Check sheet for the modelled part. Datum: model origin and axes. Units: mm. Give positions to 0.01 mm unless a question says otherwise; leave off trailing zeros. Loops run counter-clockwise (first coordinate to the right, second up) from the corner with the lowest first, then second, coordinate; pieces in that order, holes last. Notation, with made-up numbers: (-15, 10.5) -> (16, 10.5) arc R29 ccw to (16, 49.5) -> close; hole circle Ø4 at (4.5, 9). An arc over 180 degrees is marked (long way). Answer as CSV lines item,"result". Start each with the question number.
(1) Release check for a two-part mould opening along Y. For faces 1 (the face through (0.02, -6.59, 1.46)), 2 (the face through (0.02, 0.24, -20.64)), 3 (the face through (0.022, -16.642, -18.083)), 4 (the face through (-1.588, 5, -5)) record: pulls with the +Y half, pulls with the -Y half, needs draft (parallel to the pull), parting line crosses it, or undercut.
(2) Material ranges on line 1 (Y direction, x = -0.2, z = 0); line 2 (Z direction, x = 0.7, y = 5); line 3 (Y direction, x = 1, z = 4.5), recorded low to high. Write a range as from..to.
(3) Section check A-A on y = 0. Enter the section's corners in (x, z).
(4) Section check D-D on z = -13. Enter the section's corners in (x, y).
(5) Gauge pin test, flat end, axial feed: pin 1 Ø1.5 at (x, z) = (-1, -22.5) entering from -Y. Record the tip position at first contact, or that the pin passes through.
from build123d import *

# Parameters (mm, degrees)
SKETCH1_R             = 6.749999962
BOSS_EXTRUDE1_DEPTH   = 1.5875
FILLET1_R             = 0.508
FILLET2_R             = 0.508
M12_CLEARANCE_HOLE1_D = 13.5


with BuildPart() as part:
    # Sketch1 → Boss-Extrude1 (new, symmetric)
    # profile 1 of 2: a face of its own
    with BuildSketch(Plane(origin=(0, 0, 0), x_dir=(0, 0, -1), z_dir=(1, 0, 0))):
        with BuildLine():
            Line((33.3375, -12.7), (5.163771309, -19.981037814))
            ThreePointArc((5.163771309, -19.981037814), (-20.6375, 0), (5.163771309, 19.981037814))
            Line((5.163771309, 19.981037814), (33.3375, 12.7))
            ThreePointArc((33.3375, 12.7), (20.6375, 0), (33.3375, -12.7))
        make_face()
        Circle(SKETCH1_R, mode=Mode.SUBTRACT)
    # profile 2 of 2: a face of its own
    with BuildSketch(Plane(origin=(0, 0, 0), x_dir=(0, 0, -1), z_dir=(1, 0, 0))):
        Circle(SKETCH1_R)
    extrude(amount=BOSS_EXTRUDE1_DEPTH, both=True)

    # Fillet1
    fillet1_edges = [part.edges().sort_by_distance(p)[0] for p in [
        (0, -12.7, -33.3375),
    ]]
    fillet(fillet1_edges, radius=FILLET1_R)

    # Fillet2
    fillet2_edges = [part.edges().sort_by_distance(p)[0] for p in [
        (0, 12.7, -33.3375),
    ]]
    fillet(fillet2_edges, radius=FILLET2_R)

    # M12 Clearance Hole1 (through all)
    with Locations(Plane.ZY.offset(1.5875)):
        with Locations((0, 0)):
            Hole(M12_CLEARANCE_HOLE1_D / 2)


solid = part.part
Working result:
1,face 1,"undercut"
1,face 2,"undercut"
1,face 3,"pulls with the -Y half"
1,face 4,"needs draft"
2,line 1,"y = -20.64..-6.75, 6.75..20.64"
2,line 2,"z = -21.66..-4.53, 4.53..20.02"
2,line 3,"y = -20.14..-5.03, 5.03..20.14"
3,outline,"(-1.59, -20.64) -> (1.59, -20.64) -> (1.59, -6.75) -> (-1.59, -6.75) -> close; (-1.59, 6.75) -> (1.59, 6.75) -> (1.59, 20.64) -> (-1.59, 20.64) -> close"
4,outline,"(-1.59, -17.96) -> (1.59, -17.96) -> (1.59, 17.96) -> (-1.59, 17.96) -> close"
5,pin 1,"stops at y = -15.69"
